Could you check a few things on this model? Use its own coordinates, in mm. A direction names the side the tool comes from. Round coordinates to 2 decimals unless told otherwise and drop trailing zeros. Write each loop counter-clockwise with the first axis right and the second up, starting at its lowest first coordinate (ties: lowest second). Pieces come first, ordered by that corner, then holes. Notation, with made-up numbers: (80.25, 54.25) -> (135.25, 54.25) arc R27 ccw to (135.25, 89.25) -> close; hole circle Ø3 at (22.5, 12). An arc over 180 degrees is marked (long way). Answer in a Markdown table with one row per item.
from build123d import *

# Parameters (mm, degrees)
BOSS_EXTRUDE2_START     = -30
BOSS_EXTRUDE2_DEPTH     = 60
CUT_EXTRUDE1_DEPTH      = 30
CUT_EXTRUDE1_DEPTH_BACK = 12
SKETCH2_W               = 72.600000086
SKETCH2_H               = 15
CUT_EXTRUDE2_REACH      = 109.943
CUT_EXTRUDE2_END_RADIUS = 35


# Read off the part's stored shape, not the designer's step: Boss-Extrude2
with BuildPart() as part:
    # Boss-Extrude2 outline → Boss-Extrude2 (new body)
    with BuildSketch(Plane(origin=(0, 0, 0), x_dir=(1, 0, 0), z_dir=(0, 1, 0)).offset(BOSS_EXTRUDE2_START)):
        with BuildLine():
            Line((-65, 40.788), (-65, 32.788))
            Line((-65, 32.788), (-58.6640897, 32.788))
            add(Edge.make_bspline(
                [(-39.726875088, 4.666411438), (-39.726875088, 26.333078105), (-43.6640897, 32.788), (-58.6640897, 32.788)],
                knots=[0, 0, 0, 0, 1, 1, 1, 1], degree=3))
            ThreePointArc((-39.726875088, 4.666411438), (0, -40), (39.726875088, 4.666411438))
            add(Edge.make_bspline(
                [(39.726875088, 4.666411438), (39.726875088, 26.333078105), (36.335782116, 32.788), (51.335782116, 32.788)],
                knots=[0, 0, 0, 0, 1, 1, 1, 1], degree=3))
            Line((51.335782116, 32.788), (65, 32.788))
            Line((65, 32.788), (65, 40.788))
            Line((65, 40.788), (-65, 40.788))
        make_face()
        with BuildLine():
            add(Edge.make_bspline(
                [(37.322321234, 32.787999997), (37.214983937, 32.6492714), (36.601118756, 31.814611367), (35.73171702, 30.172599558), (34.800229832, 27.122418367), (34.414470427, 23.259382738), (34.438742851, 18.930468379), (34.548064386, 14.993063003), (34.641903468, 11.772708701), (34.703941427, 8.845933226), (34.725133622, 6.653478096), (34.72929314, 5.367067617), (34.727774909, 4.696007075), (34.726875088, 4.363959967)],
                knots=[0.359345427, 0.359345427, 0.359345427, 0.359345427, 0.372091813, 0.434882632, 0.49767345, 0.623255088, 0.748836725, 0.811627544, 0.874418363, 0.937209181, 0.968604591, 0.984302295, 1, 1, 1, 1], degree=3))
            ThreePointArc((34.726875088, 4.363959967), (0, -35), (-34.726875088, 4.363959967))
            add(Edge.make_bspline(
                [(-34.726875088, 4.363959967), (-34.729305052, 5.049007951), (-34.738428611, 6.435574708), (-34.793206082, 9.076539579), (-34.927377092, 12.195031477), (-35.211190541, 15.649676256), (-35.779016422, 19.912389182), (-36.900687517, 24.659444132), (-39.068630657, 29.318190534), (-41.204796111, 31.813713357), (-42.298121026, 32.787999997)],
                knots=[-0.0046531, -0.0046531, -0.0046531, -0.0046531, 0.02674231, 0.058137719, 0.120928538, 0.183719357, 0.246510175, 0.372091813, 0.49767345, 0.601270914, 0.601270914, 0.601270914, 0.601270914], degree=3))
            Line((-42.298121026, 32.787999997), (37.322321234, 32.787999997))
        make_face(mode=Mode.SUBTRACT)
    extrude(amount=BOSS_EXTRUDE2_DEPTH)

    # Sketch2 → Cut-Extrude1 (cut, two sides: drawn at the far end of the back side and taken through both)
    with BuildSketch(Plane(origin=(0, 0, 0), x_dir=(1, 0, 0), z_dir=(0, 1, 0)).offset(-CUT_EXTRUDE1_DEPTH_BACK)):
        Rectangle(SKETCH2_W, SKETCH2_H)
    extrude(amount=CUT_EXTRUDE1_DEPTH + CUT_EXTRUDE1_DEPTH_BACK, mode=Mode.SUBTRACT)

    # Cut-Extrude2: up to this cylinder (the profile starts outside it)
    cut_extrude2_end = Plane(origin=(0, 12.467931, 0), z_dir=(0, -1, 0)) * Cylinder(CUT_EXTRUDE2_END_RADIUS, 290.886, mode=Mode.PRIVATE)
    # Sketch4 → Cut-Extrude2 (cut, up to the surface)
    with BuildSketch(Plane.XY.offset(40), mode=Mode.PRIVATE) as cut_extrude2_sk1:
        with BuildLine():
            Line((7.288, 30), (7.288, 3.748))
            ThreePointArc((7.288, 3.748), (18.288, -7.252), (29.288, 3.748))
            Line((29.288, 3.748), (29.288, 30))
            Line((29.288, 30), (7.288, 30))
        make_face()
    cut_extrude2_tool1 = extrude(cut_extrude2_sk1.sketch, amount=-CUT_EXTRUDE2_REACH, mode=Mode.PRIVATE) - cut_extrude2_end
    add(cut_extrude2_tool1.solids().sort_by_distance((18.288, 12.467931, 40))[0], mode=Mode.SUBTRACT)


solid = part.part
1) For pin 1 (6 mm diameter, centred on y = 7, z = 26, fed in from -X); pin 2 (1.1 mm diameter, centred on x = 35.5, z = -2, fed in from +Y); pin 3 (4 mm diameter, centred on y = 14.5, z = 23, fed in from -X); pin 4 (8 mm diameter, centred on x = 27.5, z = -25, fed in from +Y), each with a flat end and sliding along its axis, tell me the tip position at first contact or that it passes through.
Findings:
| item | result |
|---|---|
| pin 1 | stops at x = -32.73 |
| pin 2 | stops at y = -12 |
| pin 3 | stops at x = -34.04 |
| pin 4 | passes through |
2) Thinking about a two-plate mould opening in Z: for faces 1 (the face through (65, 0, -37)), 2 (the face through (58, 0, -32.788)), 3 (the face through (-36.3, 9, 0)), 4 (the face through (0.83, -7.09, 34.99)), which applies, +Z half, -Z half, draft (parallel to the pull), parting line (faces both ways), or undercut?
Findings:
| item | result |
|---|---|
| face 1 | draft |
| face 2 | +Z half |
| face 3 | undercut |
| face 4 | undercut |
3) Imagine slicing it at C-C, the plane z = 15.5. Please give me the cut outline in (x, y).
Findings:
| item | result |
|---|---|
| outline | (-36.87, -30) -> (-31.38, -30) -> (-31.38, 30) -> (-36.87, 30) -> close; (31.38, -30) -> (36.87, -30) -> (36.87, 30) -> (31.38, 30) -> close |
4) Imagine slicing it at A-A, the plane x = 0. Please give me the cut outline in (y, z), plus the area to 3 significant figures.
Findings:
| item | result |
|---|---|
| outline | (-30, -40.79) -> (30, -40.79) -> (30, -32.79) -> (-30, -32.79) -> close; (-30, 35) -> (30, 35) -> (30, 40) -> (-30, 40) -> close |
| area | 780 mm^2 |
5) For faces 5 (the face through (36.3, 9, 0)), 6 (the face through (-3, 0, -32.788)), 7 (the face through (7.288, 17, 37)), 8 (the face through (-62, 0, -32.788)), 9 (the face through (29.288, 17, 23)), which set-ups out of +Z, -Z, +X, -X, +Y, -Y let a thin tool reach every point of the face, with its end or its side?
Findings:
| item | result |
|---|---|
| face 5 | +Y |
| face 6 | +Y, -Y |
| face 7 | +Z, +X, +Y |
| face 8 | +Z, -X, +Y, -Y |
| face 9 | +Z, +Y |
6) Imagine slicing it at B-B, the plane z = 0. Please give me the cut outline in (x, y), plus the area to 3 significant figures.
Findings:
| item | result |
|---|---|
| outline | (-40, -30) -> (-35, -30) -> (-35, -12) -> (-36.3, -12) -> (-36.3, 30) -> (-40, 30) -> close; (35, -30) -> (40, -30) -> (40, 30) -> (36.3, 30) -> (36.3, -12) -> (35, -12) -> close |
| area | 491 mm^2 |
7) Please list where these lines run through material, in increasing order: line 1 (X direction, y = -8.5, z = 0); line 2 (Y direction, x = 18, z = 35); line 3 (X direction, y = -24, z = 28.5).
Findings:
| item | result |
|---|---|
| line 1 | x = -40 to -36.3, 36.3 to 40 |
| line 2 | y = -30 to -7.25 |
| line 3 | x = -28.07 to -20.32, 20.32 to 28.07 |
